Part model, mm, in its own coordinate system. Round coordinates to 2 decimals unless told otherwise and drop trailing zeros. Write each loop counter-clockwise with the first axis right and the second up, starting at its lowest first coordinate (ties: lowest second). Pieces come first, ordered by that corner, then holes. Notation, with made-up numbers: M -5.5,-21.5 L 49.5,-21.5 A15 cw 49.5,-5.5 Z; hole C 18.25,24.25 d7. An arc over 180 degrees is marked long. Use a Markdown table: item, result. Add a question column.
1) Slice it at A-A on z = 32. Write the cut outline in (x, y).
2) Drop a flat-ended pin along its axis: P1, Ø3, axis at x = -53.5, y = -3.5, coming from the -Z side. Give the stop position or say it passes through.
3) Wall check: probe 1 along Z at (x, y) = (-52.75, -3); probe 2 along Z at (x, y) = (-51.25, -5.25); probe 3 along X at (y, z) = (-1.5, 53). Give the ranges that are in metal, low to high.
4) Slice it at D-D on z = 18. Write the cut outline in (x, y).
5) Two-plate mould, pull along X, no slides. Class faces 1 (the face through (-58.78, -3.22, -5.8)), 2 (the face through (-50.945, -3.131, 65.597)), 3 (the face through (-38.522, -3, 26)): released by +X, released by -X, zero draft, split by the parting line, or undercut.
6) Slice it at B-B on y = -0.75. Write the cut outline in (x, z) (3 decimals), plus the area to 3 significant figures.
7) Slice it at C-C on x = -48.75. Write the cut outline in (y, z), plus the area to 3 significant figures.
```python
from build123d import *

# Parameters (mm, degrees)
F1_DEPTH = 6.35
F2_R     = 9.525
F3_DEPTH = 25.4


with BuildPart() as f1:
    # F0 (on Front) → F1 (new body)
    with BuildSketch(Plane.XZ):
        with BuildLine():
            ThreePointArc((-38.521796, 52.898269), (-51.223841, 65.600313), (-63.925885, 52.898269))
            Line((-63.925885, 52.898269), (-63.925885, 0))
            ThreePointArc((-63.925885, 0), (-51.223841, -12.702044), (-38.521796, 0))
            Line((-38.521796, 0), (-38.521796, 52.898269))
        make_face()
    extrude(amount=F1_DEPTH)

    # F2 (on face) → F3 (cut)
    with BuildSketch(Plane.XZ.offset(6.35)):
        with Locations((-51.223841, 24.542077)):
            Circle(F2_R)
        with Locations((-51.223841, 0)):
            Circle(F2_R)
        with Locations((-51.223841, 52.898269)):
            Circle(F2_R)
    extrude(amount=-F3_DEPTH, mode=Mode.SUBTRACT)


solid = f1.part
```
Entries:
| question | item | result |
|---|---|---|
| 1 | outline | M -63.93,-6.35 L -57.15,-6.35 L -57.15,0 L -63.93,0 Z; M -45.3,-6.35 L -38.52,-6.35 L -38.52,0 L -45.3,0 Z |
| 2 | P1 | stops at z = -12.68 |
| 3 | probe 1 | z = -12.61 to -9.4, 9.4 to 15.14, 33.94 to 43.5, 62.3 to 65.51 |
| 3 | probe 2 | z = -12.7 to -9.52, 9.52 to 15.02, 34.07 to 43.37, 62.42 to 65.6 |
| 3 | probe 3 | x = -63.93 to -60.75, -41.7 to -38.52 |
| 4 | outline | M -63.93,-6.35 L -58.15,-6.35 L -58.15,0 L -63.93,0 Z; M -44.3,-6.35 L -38.52,-6.35 L -38.52,0 L -44.3,0 Z |
| 5 | face 1 | undercut |
| 5 | face 2 | split by the parting line |
| 5 | face 3 | released by +X |
| 6 | outline | M -63.926,0 A12.702 ccw -38.522,0 L -38.522,52.898 A12.702 ccw -63.926,52.898 Z; hole C -51.224,0 d19.05; hole C -51.224,24.542 d19.05; hole C -51.224,52.898 d19.05 |
| 6 | area | 996 mm^2 |
| 7 | outline | M -6.35,-12.46 L 0,-12.46 L 0,-9.2 L -6.35,-9.2 Z; M -6.35,9.2 L 0,9.2 L 0,15.34 L -6.35,15.34 Z; M -6.35,33.74 L 0,33.74 L 0,43.7 L -6.35,43.7 Z; M -6.35,62.1 L 0,62.1 L 0,65.36 L -6.35,65.36 Z |
| 7 | area | 144 mm^2 |
